Study the drawing (mm; zero at the part's minimum x, y, z) and answer. A direction names the side the tool comes from. Coordinates: 2 decimals unless noted, no trailing zeros. Order: outer loops, then holes, each group sorted by start corner. A loop starts at its lowest first (then second) coordinate and runs counter-clockwise, first axis right, second up.
1. Determine the mould class of the marked faces 3, 4, 5 and 6 for opening direction Z: +Z half, -Z half, draft (parallel to the pull), parting line (faces both ways), or undercut.
2. A tool of negligible diameter and unlimited length cuts with its end or side. For the marked faces 1 and 2, from which of +Z, -Z, +X, -X, +Y, -Y can it reach the whole face along a straight path? Write none if from no direction.
3. Flat-ended cylindrical pins translate along their axes: pin 1 Ø1 at (x, y) = (36.5, 9) entering from -Z; pin 2 Ø8 at (y, z) = (5.5, 15.5) entering from +X. Find the tip coordinate at first contact, or state that the pin passes through.
4. Find the intervals of material crossed by probe 1 along Z at (x, y) = (39.5, 10.25); probe 2 along X at (y, z) = (9.25, 31); probe 3 along Y at (x, z) = (25.5, 23), in increasing order.
5. The part is cut by section C-C, the plane z = 10.5. Give the vertices of the cut face in (x, y).
6. The part is cut by section B-B, the plane x = 32.5. Give the vertices of the cut face in (y, z).
7. The part is cut by section A-A, the plane y = 2.25. Give the vertices of the cut face in (x, z).
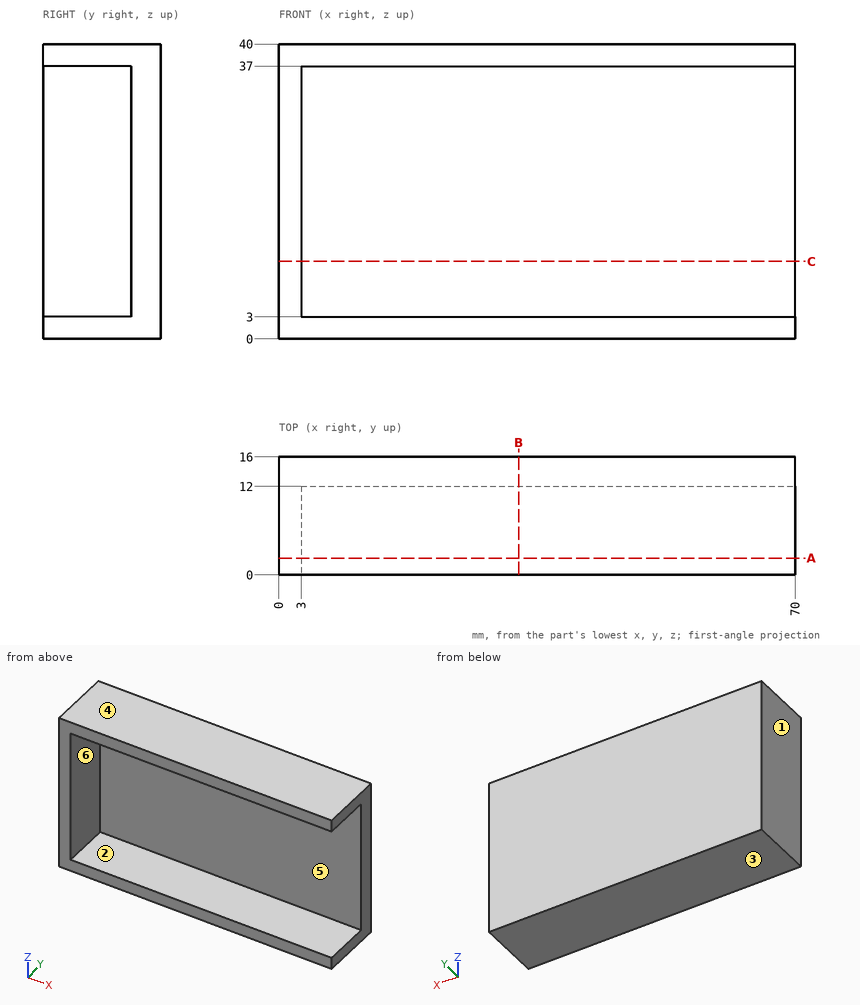
Geometry says:
1. face 3: -Z half
1. face 4: +Z half
1. face 5: undercut
1. face 6: undercut
2. face 1: +Z, -Z, -X, +Y, -Y
2. face 2: +X, -Y
3. pin 1: stops at z = 0
3. pin 2: stops at x = 3
4. probe 1: z = 0 to 3, 37 to 40
4. probe 2: x = 0 to 3
4. probe 3: y = 12 to 16
5. outline: (0, 0) - (3, 0) - (3, 12) - (70, 12) - (70, 16) - (0, 16) - close
6. outline: (0, 0) - (16, 0) - (16, 40) - (0, 40) - (0, 37) - (12, 37) - (12, 3) - (0, 3) - close
7. outline: (0, 0) - (70, 0) - (70, 3) - (3, 3) - (3, 37) - (70, 37) - (70, 40) - (0, 40) - close
